Source: CAD feature listing. Evaluate the final solid. Frame: model axes, mm. Face numbers are marked on the shaded views. Coordinates: 2 decimals unless noted, no trailing zeros. Write each loop counter-clockwise with the first axis right and the second up, starting at its lowest first coordinate (ties: lowest second). Pieces come first, ordered by that corner, then holes. Notation, with made-up numbers: (24, 70.25) - (81, 70.25) arc R24 cw to (81, 109.25) - close; hole circle Ø10 at (85.5, 30). An arc over 180 degrees is marked (long way). One line per question, with ' | ' between items. Start each with the question number.
Q1. Draft query along Z for the marked faces 1, 2, 3 and 4. Return one class per face: +Z half, -Z half, draft (parallel to the pull), parting line (faces both ways), or undercut.
Q2. Cut plane D-D, the plane x = -45. Return loops of the section in (y, z), plus the area to 3 significant figures.
Q3. Cut plane A-A, the plane y = 0. Return loops of the section in (x, z), plus the area to 3 significant figures.
Q4. Cut plane B-B, the plane y = -35. Return loops of the section in (x, z), plus the area to 3 significant figures.
Q5. Cut plane C-C, the plane z = -25.5. Return loops of the section in (x, y), plus the area to 3 significant figures.
Q6. Line query: line 1 (Y direction, x = 0, z = -34); line 2 (Y direction, x = 0, z = -18.5); line 3 (Z direction, x = -44.5, y = -39.5). Output: solid intervals per line, ascending.
Q7. Contact query for flat-ended pins moving along their axis: P1, Ø1.5, axis at x = 47, z = -24.5, coming from the -Y side; P2, Ø13.5, axis at x = 0, y = 35, coming from the +Z side; P3, Ø12, axis at x = 14.5, z = -26, coming from the +Y side; P4, Ø10, axis at x = 16.5, y = 44.5, coming from the -Z side. Output: stop coordinate, or through.
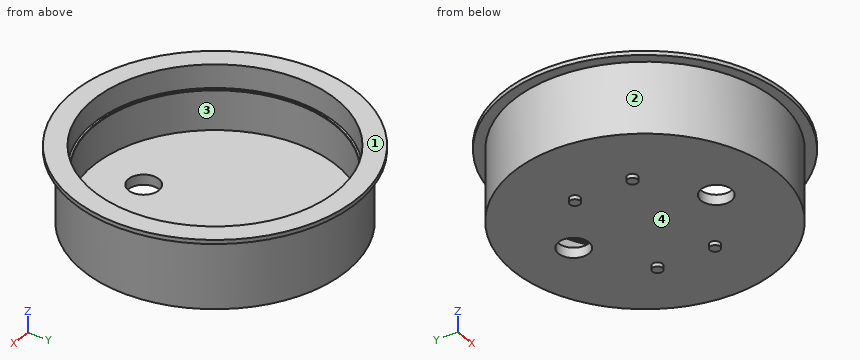
```python
from build123d import *

# Parameters (mm, degrees)
F0_R      = 70
F1_DEPTH  = 2
F2_R      = 65
F3_DEPTH  = 35
F4_R      = 60
F5_DEPTH  = 32
F6_R      = 7.5
F7_DEPTH  = 5.001
F8_R      = 2.5
F9_DEPTH  = 2
F11_R     = 62.2
F11_R_2   = 59
F12_DEPTH = 0.5


with BuildPart() as f1:
    # F0 (on Top) → F1 (new body)
    with BuildSketch(Plane.XY):
        Circle(F0_R)
    extrude(amount=-F1_DEPTH)

    # F2 (on face) → F3 (join)
    with BuildSketch(Plane(origin=(0, 0, -2), x_dir=(1, 0, 0), z_dir=(0, 0, -1))):
        Circle(F2_R)
    extrude(amount=F3_DEPTH)

    # F4 (on face) → F5 (cut)
    with BuildSketch(Plane.XY):
        Circle(F4_R)
    extrude(amount=-F5_DEPTH, mode=Mode.SUBTRACT)

    # F6 (on face) → F7 (cut, through all)
    with BuildSketch(Plane.XY.offset(-32)):
        with Locations((0, -35)):
            Circle(F6_R)
        with Locations((0, 35)):
            Circle(F6_R)
    extrude(amount=-F7_DEPTH, mode=Mode.SUBTRACT)

    # F8 (on face) → F9 (join)
    with BuildSketch(Plane(origin=(0, 0, -37), x_dir=(1, 0, 0), z_dir=(0, 0, -1))):
        with Locations((-30, 14.127)):
            Circle(F8_R)
        with Locations((-30, -14.12747)):
            Circle(F8_R)
        with Locations((30, 14.127)):
            Circle(F8_R)
        with Locations((30, -14.12747)):
            Circle(F8_R)
    extrude(amount=F9_DEPTH)

    # F11 (on offset) → F12 (join)
    with BuildSketch(Plane.XY.offset(-12)):
        Circle(F11_R)
        Circle(F11_R_2, mode=Mode.SUBTRACT)
    extrude(amount=F12_DEPTH)


solid = f1.part
```
Reply:
1) face 1: +Z half | face 2: draft | face 3: undercut | face 4: -Z half
2) outline: (-53.62, -2) - (-46.9, -2) - (-46.9, -37) - (46.9, -37) - (46.9, -2) - (53.62, -2) - (53.62, 0) - (39.69, 0) - (39.69, -11.5) - (38.16, -11.5) - (38.16, -12) - (39.69, -12) - (39.69, -32) - (-39.69, -32) - (-39.69, -12) - (-38.16, -12) - (-38.16, -11.5) - (-39.69, -11.5) - (-39.69, 0) - (-53.62, 0) - close | area: 959 mm^2
3) outline: (-70, -2) - (-65, -2) - (-65, -37) - (65, -37) - (65, -2) - (70, -2) - (70, 0) - (60, 0) - (60, -11.5) - (59, -11.5) - (59, -12) - (60, -12) - (60, -32) - (-60, -32) - (-60, -12) - (-59, -12) - (-59, -11.5) - (-60, -11.5) - (-60, 0) - (-70, 0) - close | area: 991 mm^2
4) outline: (-60.62, -2) - (-54.77, -2) - (-54.77, -37) - (-7.5, -37) - (-7.5, -32) - (-48.73, -32) - (-48.73, -12) - (-47.5, -12) - (-47.5, -11.5) - (-48.73, -11.5) - (-48.73, 0) - (-60.62, 0) - close; (7.5, -37) - (54.77, -37) - (54.77, -2) - (60.62, -2) - (60.62, 0) - (48.73, 0) - (48.73, -11.5) - (47.5, -11.5) - (47.5, -12) - (48.73, -12) - (48.73, -32) - (7.5, -32) - close | area: 884 mm^2
5) outline: circle Ø130 at (0, 0); hole circle Ø120 at (0, 0) | area: 1,960 mm^2
6) line 1: y = -65 to -42.5, -27.5 to 27.5, 42.5 to 65 | line 2: y = -65 to -60, 60 to 65 | line 3: z = -37 to -32, -12 to -11.5
7) P1: stops at y = -45.67 | P2: passes through | P3: stops at y = 64.44 | P4: stops at z = -37
